```python
from build123d import *

# Parameters (mm, degrees)
F0_R     = 4.3560889736
F1_DEPTH = 50.8


with BuildPart() as f1:
    # F0 (on Front) → F1 (new body)
    with BuildSketch(Plane.XZ):
        with BuildLine():
            ThreePointArc((-50.8035481042, 44.8743139746), (-37.3327925125, 20.3368670349), (-15.7611440911, 38.1753519177))
            ThreePointArc((-15.7611440911, 38.1753519177), (-23.931762198, 53.3418471705), (-41.0919163358, 54.8619420575))
            Line((-41.0919163358, 54.8619420575), (-40.6960048204, 54.4206382187))
            Line((-40.6960048204, 54.4206382187), (-39.7726875247, 51.561406541))
            Line((-39.7726875247, 51.561406541), (-40.0921494975, 48.5738214521))
            Line((-40.0921494975, 48.5738214521), (-41.5991528616, 45.9744635553))
            Line((-41.5991528616, 45.9744635553), (-44.0331230447, 44.2127854453))
            Line((-44.0331230447, 44.2127854453), (-46.97320449, 43.5933972717))
            Line((-46.97320449, 43.5933972717), (-49.9110304061, 44.2233968767))
            Line((-49.9110304061, 44.2233968767), (-50.8035481042, 44.8743139746))
        make_face()
        with Locations((-29.9666635692, 36.7907546461)):
            Circle(F0_R, mode=Mode.SUBTRACT)
        with BuildLine():
            Line((-40.6960048204, 54.4206382187), (-41.0919163358, 54.8619420575))
            ThreePointArc((-41.0919163358, 54.8619420575), (-46.9434332236, 50.8363139975), (-50.8035481042, 44.8743139746))
            Line((-50.8035481042, 44.8743139746), (-49.9110304061, 44.2233968767))
            Line((-49.9110304061, 44.2233968767), (-46.97320449, 43.5933972717))
            Line((-46.97320449, 43.5933972717), (-44.0331230447, 44.2127854453))
            Line((-44.0331230447, 44.2127854453), (-41.5991528616, 45.9744635553))
            Line((-41.5991528616, 45.9744635553), (-40.0921494975, 48.5738214521))
            Line((-40.0921494975, 48.5738214521), (-39.7726875247, 51.561406541))
            Line((-39.7726875247, 51.561406541), (-40.6960048204, 54.4206382187))
        make_face()
        with BuildLine():
            ThreePointArc((-50.8035481042, 44.8743139746), (-46.9434332236, 50.8363139975), (-41.0919163358, 54.8619420575))
            Line((-41.0919163358, 54.8619420575), (-42.7024514363, 56.6571293527))
            Line((-42.7024514363, 56.6571293527), (-45.4450945244, 57.8841703083))
            Line((-45.4450945244, 57.8841703083), (-48.4497061786, 57.8895945568))
            Line((-48.4497061786, 57.8895945568), (-51.1967617479, 56.6724641964))
            Line((-51.1967617479, 56.6724641964), (-53.2112703682, 54.4432321237))
            Line((-53.2112703682, 54.4432321237), (-54.1449051977, 51.587352816))
            Line((-54.1449051977, 51.587352816), (-53.8362322927, 48.5986337504))
            Line((-53.8362322927, 48.5986337504), (-52.3386240026, 45.9938516051))
            Line((-52.3386240026, 45.9938516051), (-50.8035481042, 44.8743139746))
        make_face()
    extrude(amount=F1_DEPTH)


solid = f1.part
```
The listing builds one solid part. Answer for the finished solid, in the listing's coordinates (mm). A direction names the side the tool comes from. Coordinates: 2 decimals unless noted, no trailing zeros. Write each loop counter-clockwise with the first axis right and the second up, starting at its lowest first coordinate (ties: lowest second). Pieces come first, ordered by that corner, then holes. Notation, with made-up numbers: (6.25, -31.75) - (13.25, -31.75) arc R20 cw to (13.25, -27.75) - close; hole circle Ø6 at (87.5, 22.5). An arc over 180 degrees is marked (long way). Return JSON: item names as keys, results as strings. Group by question number.
Q1. The part is cut by section C-C on z = 40. Write down the section's boundary in (x, y).
Q2. Find the intervals of material crossed by line 1 along Z through (x, y) = (-28, -41); line 2 along Z through (x, y) = (-33, -17); line 3 along X through (y, z) = (-40, 38.5), in increasing order. Write a range as [from, to].
Q3. For a pull along X with two mould halves and no side action, classify faces 1 (the flat face through (-41.89, -25.04, 55.75)), 2 (the flat face through (-35, 0, 39)), 3 (the flat face through (-53.67, -25.04, 53.04)) as +X half, -X half, draft (parallel to the pull), parting line (faces both ways), or undercut.
Q4. The part is cut by section D-D on x = -47. Write down the section's boundary in (y, z).
Q5. Which of the six approach directions +Z, -Z, +X, -X, +Y, -Y give full straight-line access (tool end or side, diameter ignored) to faces 4 (the flat face through (-35, -50.8, 39)), 5 (the flat face through (-51.58, -25.04, 45.44))?
Q6. The part is cut by section A-A on x = -33.5. Write down the section's boundary in (y, z).
Q7. Flat-ended cylindrical pins translate along their axes: pin 1 Ø8 at (x, z) = (-29.97, 36.79) entering from -Y; pin 2 Ø3 at (y, z) = (-33.5, 28) entering from +X; pin 3 Ø1.5 at (y, z) = (-25, 25.5) entering from -X; pin 4 Ø6 at (y, z) = (-14, 43) entering from +X. Find the tip coordinate at first contact, or state that the pin passes through.
Q8. The part is cut by section B-B on y = -7.5. Write down the section's boundary in (x, z), and give its area (3 significant figures).
Evaluation:
{
 "1": {"outline": "(-51.99, -50.8) - (-32.91, -50.8) - (-32.91, 0) - (-51.99, 0) - close; (-27.02, -50.8) - (-15.85, -50.8) - (-15.85, 0) - (-27.02, 0) - close"},
 "2": {"line 1": "z = [21.01, 32.9], [40.68, 55.34]", "line 2": "z = [20.04, 33.66], [39.92, 56.31]", "line 3": "x = [-52.08, -33.97], [-25.96, -15.76]"},
 "3": {"face 1": "undercut", "face 2": "draft", "face 3": "-X half"},
 "4": {"outline": "(-50.8, 25.57) - (0, 25.57) - (0, 57.89) - (-50.8, 57.89) - close"},
 "5": {"face 4": "+Z, -Z, +X, -X, -Y", "face 5": "-X, +Y, -Y"},
 "6": {"outline": "(-50.8, 20.02) - (0, 20.02) - (0, 34.24) - (-50.8, 34.24) - close; (-50.8, 39.34) - (0, 39.34) - (0, 56.33) - (-50.8, 56.33) - close"},
 "7": {"pin 1": "passes through", "pin 2": "stops at x = -17.97", "pin 3": "stops at x = -47.62", "pin 4": "stops at x = -15.85"},
 "8": {"outline": "(-54.14, 51.59) - (-53.84, 48.6) - (-52.34, 45.99) - (-50.8, 44.87) arc R18.16 ccw (long way) to (-41.09, 54.86) - (-42.7, 56.66) - (-45.45, 57.88) - (-48.45, 57.89) - (-51.2, 56.67) - (-53.21, 54.44) - close; hole circle Ø8.71 at (-29.97, 36.79)", "area": "1,060 mm2"}
}
